Here's the drawing with two shaded views (mm, measured from the low corner). I have some questions. Coordinates: 2 decimals unless noted, no trailing zeros. Loops run counter-clockwise (first coordinate to the right, second up) from the corner with the lowest first, then second, coordinate; pieces in that order, holes last. Notation, with made-up numbers: (-26, 71.5) - (-3, 71.5) arc R27 cw to (-3, 98.5) - close; hole circle Ø11 at (74, -26.5). An arc over 180 degrees is marked (long way). One line per item, written item: value. Start each with the question number.
(1) If we section it at A-A on z = 41: Write out the boundary of the cut face in (x, y).
(2) If we mould it in two halves opening along Z, with no side actions, what happens to the marked faces 1 and 2? For each: pulls with the +Z half, pulls with the -Z half, needs draft (parallel to the pull), parting line crosses it, or undercut.
(3) If we section it at C-C on x = 2.5: Write out the boundary of the cut face in (y, z).
(4) If I drill on line 1 along Y through (x, z) = (2.3, 41); line 2 along Z through (x, y) = (2.75, 44.5); line 3 along Y through (x, z) = (2.2, 46), over which ranges is the centre line in solid material (lowest first)? Write a range as from..to.
(5) If we section it at B-B on y = 44: Write out the boundary of the cut face in (x, z).
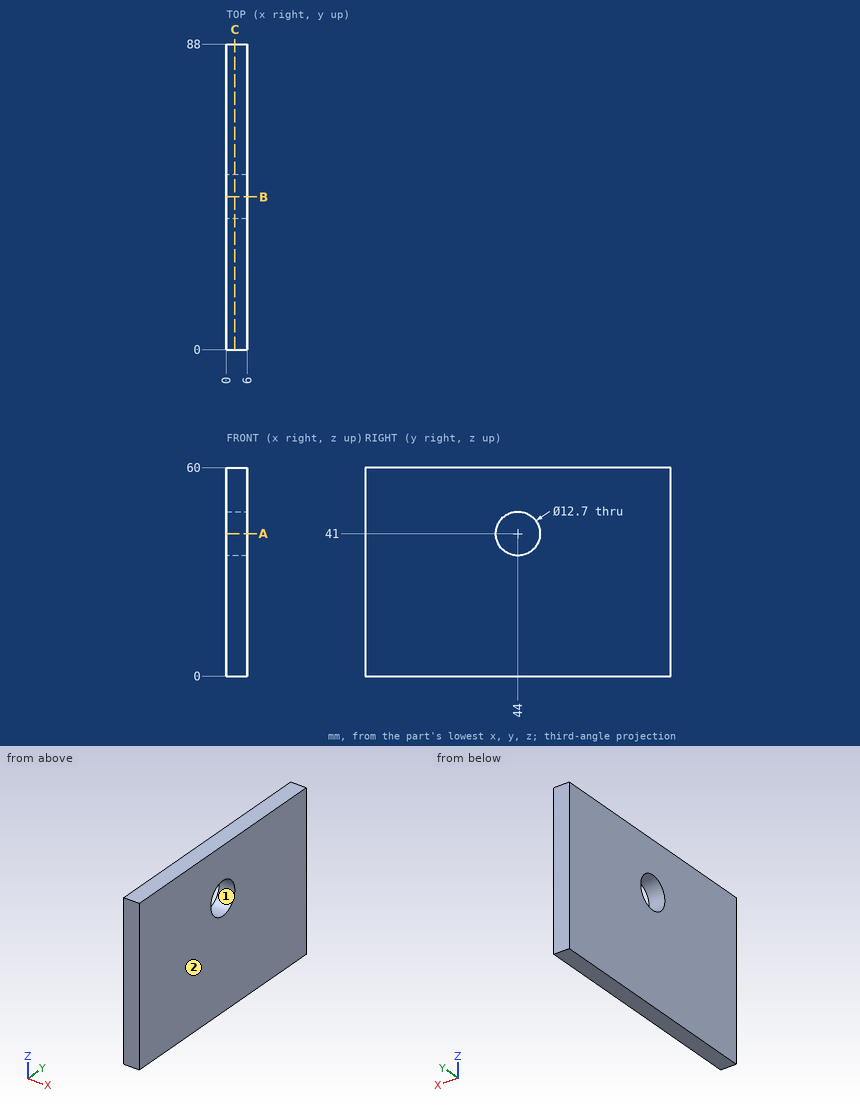
Values:
1. outline: (0, 0) - (6, 0) - (6, 37.65) - (0, 37.65) - close; (0, 50.35) - (6, 50.35) - (6, 88) - (0, 88) - close
2. face 1: undercut
2. face 2: needs draft
3. outline: (0, 0) - (88, 0) - (88, 60) - (0, 60) - close; hole circle Ø12.7 at (44, 41)
4. line 1: y = 0..37.65, 50.35..88
4. line 2: z = 0..34.67, 47.33..60
4. line 3: y = 0..40.09, 47.91..88
5. outline: (0, 0) - (6, 0) - (6, 34.65) - (0, 34.65) - close; (0, 47.35) - (6, 47.35) - (6, 60) - (0, 60) - close
